The model under review builds one solid part; all positions refer to its coordinate system, in mm. A direction names the side the tool comes from. Round coordinates to 2 decimals unless told otherwise and drop trailing zeros. Loops run counter-clockwise (first coordinate to the right, second up) from the corner with the lowest first, then second, coordinate; pieces in that order, holes last. Notation, with made-up numbers: M -1.5,19.25 L 16.5,19.25 A22 cw 16.5,51.25 Z; hole C -19,58 d5. An arc over 180 degrees is marked long. Answer as a JSON object with one key per item and string values. Group by question number.
Item 1: Consider section B-B (y = -7). Give the boundary of the cut face in (x, z), and give its area (3 significant figures).
Item 2: Consider section D-D (x = 123). Give the boundary of the cut face in (y, z).
Item 3: Consider section A-A (z = 176.5). Give the boundary of the cut face in (x, y), and give its area (3 significant figures).
Item 4: To check wall thickness, follow line 1 (Z direction, x = 81, y = -5); line 2 (X direction, y = -70, z = 174.5); line 3 (X direction, y = -69, z = -14). State the ranges of each line that lie inside material, in increasing order.
Item 5: Consider section C-C (x = 4). Give the boundary of the cut face in (y, z), and give its area (3 significant figures).
Item 6: Insertion check: P1, Ø2, axis at x = 25.5, y = -12.5, coming from the -Z side; P2, Ø6, axis at y = -67, z = 13.5, coming from the +X side; P3, Ø1, axis at x = -60.5, z = 248.5, coming from the -Y side. Each pin has a flat end and moves straight along its axis. Give the tip position at first contact, or say it passes through.
Item 7: The part is to be moulded in two halves that separate along X. For faces 5 (the face through (-101.05, -49.92, 19.96)), 6 (the face through (-70.85, -77.69, 239.99)), 7 (the face through (-130, -49, -34)), say which applies: +X half, -X half, draft (parallel to the pull), parting line (faces both ways), or undercut.
Item 8: Tool access review of faces 1 (the face through (-120, -78, 0)), 2 (the face through (-120, -22, 0)), 3 (the face through (-83.01, -49.3, 228.15)), 4 (the face through (-64.99, -78.31, 2.85)): name each direction out of +Z, -Z, +X, -X, +Y, -Y from which nothing blocks a thin tool from reaching the whole face with its end or side.
```python
from build123d import *

# Parameters (mm, degrees)
F1_DEPTH = 100
F2_R     = 12.5
F3_DEPTH = 100
F4_R     = 5
F7_DEPTH = 6
F8_R     = 10


with BuildPart() as f1:
    # F0 (on Front) → F1 (new body)
    with BuildSketch(Plane.XZ):
        Polygon((-150, 0), (-150, -44), (-130, -44), (-130, -24), (130, -24), (130, -44), (150, -44), (150, 0), align=None)
    extrude(amount=F1_DEPTH)

    # F2 (on Front) → F3 (join)
    with BuildSketch(Plane.XZ):
        with BuildLine():
            Line((-80, 221), (-80, 0))
            Line((-80, 0), (-68, 0))
            Line((-68, 0), (-68, 233))
            ThreePointArc((-68, 233), (-70.9289321881, 240.0710678119), (-78, 243))
            Line((-78, 243), (-108.6458434959, 243))
            ThreePointArc((-108.6458434959, 243), (-117.7525512861, 234.2055052823), (-130, 231))
            Line((-130, 231), (-90, 231))
            ThreePointArc((-90, 231), (-82.9289321881, 228.0710678119), (-80, 221))
        make_face()
        with BuildLine():
            ThreePointArc((-105, 256), (-147.6776695297, 273.6776695297), (-130, 231))
            ThreePointArc((-130, 231), (-117.7525512861, 234.2055052823), (-108.6458434959, 243))
            ThreePointArc((-108.6458434959, 243), (-105.9287109547, 249.2492190304), (-105, 256))
        make_face()
        with Locations((-130, 256)):
            Circle(F2_R, mode=Mode.SUBTRACT)
    extrude(amount=F3_DEPTH)

    # F4
    f4_edges = [f1.edges().sort_by_distance(p)[0] for p in [
        (-108.645843, -50, 243),
    ]]
    fillet(f4_edges, radius=F4_R)

    # F6 (on offset) → F7 (join, symmetric)
    with BuildSketch(Plane(origin=(0, -50, 0), x_dir=(-1, 0, 0), z_dir=(0, 1, 0))):
        with BuildLine():
            ThreePointArc((105.9052795087, 249.3333333333), (110.1044393561, 271.1382517705), (130, 281))
            Line((130, 281), (40, 281))
            ThreePointArc((40, 281), (-9.4974746831, 260.4974746831), (-30, 211))
            Line((-30, 211), (-30, 70))
            ThreePointArc((-30, 70), (-50.5025253169, 20.5025253169), (-100, 0))
            Line((-100, 0), (68, 0))
            Line((68, 0), (68, 233))
            ThreePointArc((68, 233), (70.9289321881, 240.0710678119), (78, 243))
            Line((78, 243), (101.0863354104, 243))
            ThreePointArc((101.0863354104, 243), (105.0654475392, 244.9723496459), (105.9052795087, 249.3333333333))
        make_face()
        with BuildLine():
            ThreePointArc((150, 0), (100.5025253169, 20.5025253169), (80, 70))
            Line((80, 70), (80, 0))
            Line((80, 0), (150, 0))
        make_face()
    extrude(amount=F7_DEPTH, both=True)

    # F8
    f8_edges = [f1.edges().sort_by_distance(p)[0] for p in [
        (-80, -78, 0),
        (-80, -22, 0),
        (-68, -22, 0),
        (-68, -78, 0),
    ]]
    fillet(f8_edges, radius=F8_R)


solid = f1.part
```
Geometry results:
{
 "1": {"outline": "M -150,-44 L -130,-44 L -130,-24 L 130,-24 L 130,-44 L 150,-44 L 150,0 L -58,0 A10 cw -68,10 L -68,233 A10 ccw -78,243 L -101.09,243 A5 cw -105.91,249.33 A25 ccw long -130,231 L -90,231 A10 cw -80,221 L -80,10 A10 cw -90,0 L -150,0 Z; hole C -130,256 d25", "area": "12,900 mm^2"},
 "2": {"outline": "M -100,-24 L 0,-24 L 0,0 L -100,0 Z"},
 "3": {"outline": "M -80,-100 L -68,-100 L -68,-56 L 30,-56 L 30,-44 L -68,-44 L -68,0 L -80,0 Z", "area": "2,380 mm^2"},
 "4": {"line 1": "z = -24 to 0", "line 2": "x = -80 to -68", "line 3": "x = -150 to 150"},
 "5": {"outline": "M -100,-24 L 0,-24 L 0,0 L -44,0 L -44,265.44 L -56,265.44 L -56,0 L -100,0 Z", "area": "5,590 mm^2"},
 "6": {"P1": "stops at z = -24", "P2": "stops at x = -68", "P3": "stops at y = -56"},
 "7": {"face 5": "-X half", "face 6": "+X half", "face 7": "undercut"},
 "8": {"face 1": "-X, -Y", "face 2": "-X, +Y", "face 3": "-X, +Y, -Y", "face 4": "+Z, +X, -Y"}
}
